```python
from build123d import *

# Parameters (mm, degrees)
SKETCH3_W           = 18.934254216
SKETCH3_H           = 5
BOSS_EXTRUDE1_DEPTH = 8
CUT_EXTRUDE1_REACH  = 24.954
SKETCH5_R           = 1.05
SKETCH4_W           = 5.27
SKETCH4_H           = 5
CUT_EXTRUDE2_DEPTH  = 2.9
SKETCH6_W           = 5.27
SKETCH6_H           = 5
CUT_EXTRUDE3_DEPTH  = 5.4
CUT_EXTRUDE5_REACH  = 15.365
CUT_EXTRUDE6_REACH  = 24.954
SKETCH10_R          = 1.7
CUT_EXTRUDE9_DEPTH  = 2
FILLET1_R           = 2.5
FILLET2_R           = 1.75
CUT_EXTRUDE7_REACH  = 15.365
SKETCH8_W           = 3.025341734
SKETCH8_H           = 1.75
CHAMFER1_SIZE       = 1


with BuildPart() as part:
    # Sketch3 → Boss-Extrude1 (new body)
    with BuildSketch(Plane.ZY):
        with Locations((0, 16.820132754)):
            Rectangle(SKETCH3_W, SKETCH3_H)
    extrude(amount=-BOSS_EXTRUDE1_DEPTH)

    # Sketch5 → Cut-Extrude1 (cut, up to next)
    with BuildSketch(Plane.ZY, mode=Mode.PRIVATE) as cut_extrude1_sk1:
        with Locations(Location((6.967127108, 16.820132754, 0), (0, 0, 270))):
            Circle(SKETCH5_R)
    cut_extrude1_tool1 = extrude(cut_extrude1_sk1.sketch, amount=-CUT_EXTRUDE1_REACH, mode=Mode.PRIVATE) & part.part
    # Sketch5 → Cut-Extrude1 (cut, up to next)
    with BuildSketch(Plane.ZY, mode=Mode.PRIVATE) as cut_extrude1_sk2:
        with Locations(Location((-6.967127108, 16.820132754, 0), (0, 0, 270))):
            Circle(SKETCH5_R)
    cut_extrude1_tool2 = extrude(cut_extrude1_sk2.sketch, amount=-CUT_EXTRUDE1_REACH, mode=Mode.PRIVATE) & part.part
    add(cut_extrude1_tool1.solids().sort_by_distance((0, 16.820133, 6.967127))[0], mode=Mode.SUBTRACT)
    add(cut_extrude1_tool2.solids().sort_by_distance((0, 16.820133, -6.967127))[0], mode=Mode.SUBTRACT)

    # Sketch4 → Cut-Extrude2 (cut)
    with BuildSketch(Plane.ZY):
        with Locations((6.832127108, 16.820132754)):
            Rectangle(SKETCH4_W, SKETCH4_H)
    extrude(amount=-CUT_EXTRUDE2_DEPTH, mode=Mode.SUBTRACT)

    # Sketch6 → Cut-Extrude3 (cut)
    with BuildSketch(Plane(origin=(8, 0, 0), x_dir=(0, 0, -1), z_dir=(1, 0, 0))):
        with Locations((6.832127108, 16.820132754)):
            Rectangle(SKETCH6_W, SKETCH6_H)
    extrude(amount=-CUT_EXTRUDE3_DEPTH, mode=Mode.SUBTRACT)

    # Sketch1 → Cut-Extrude5 (cut, up to next)
    with BuildSketch(Plane(origin=(0, 14.320132754, 0), x_dir=(-1, 0, 0), z_dir=(0, -1, 0)), mode=Mode.PRIVATE) as cut_extrude5_sk1:
        Polygon((3.959797975, 0), (0, -3.959797975), (-3.959797975, 0), (0, 3.959797975), align=None)
    cut_extrude5_tool1 = extrude(cut_extrude5_sk1.sketch, amount=-CUT_EXTRUDE5_REACH, mode=Mode.PRIVATE) & part.part
    add(cut_extrude5_tool1.solids().sort_by_distance((0, 14.320133, 0))[0], mode=Mode.SUBTRACT)

    # Sketch7 → Cut-Extrude6 (cut, up to next)
    with BuildSketch(Plane.ZY, mode=Mode.PRIVATE) as cut_extrude6_sk1:
        Polygon((-4.197127108, 17.820132754), (4.197127108, 17.820132754), (5.697127108, 19.320132754), (-5.697127108, 19.320132754), align=None)
    cut_extrude6_tool1 = extrude(cut_extrude6_sk1.sketch, amount=-CUT_EXTRUDE6_REACH, mode=Mode.PRIVATE) & part.part
    add(cut_extrude6_tool1.solids().sort_by_distance((0, 18.608034, 0))[0], mode=Mode.SUBTRACT)

    # Sketch10 → Cut-Extrude9 (cut)
    with BuildSketch(Plane(origin=(8, 0, 0), x_dir=(0, 0, -1), z_dir=(1, 0, 0))):
        with Locations(Location((-6.967127108, 16.820132754, 0), (0, 0, 90))):
            Circle(SKETCH10_R)
    extrude(amount=-CUT_EXTRUDE9_DEPTH, mode=Mode.SUBTRACT)

    # Mirror2: part across plane


with BuildPart() as part_1:
    add(part.part)
    add(part.part.mirror(Plane(origin=(0, 0, 0), x_dir=(0, 0, 1), z_dir=(1, 0, 0))))

    # Fillet1
    # the kernel refuses this fillet: 2.5 mm, written as the material it takes off along each edge
    with BuildSketch(Plane(origin=(3.35, 14.320132754, 9.467127108), x_dir=(0, 0, -1), z_dir=(-1, 0, 0)), Plane(origin=(-3.35, 19.320132754, 9.467127108), x_dir=(0, 0, -1), z_dir=(1, 0, 0))) as fillet1_piece_1:
        with BuildLine():
            CenterArc((FILLET1_R, -FILLET1_R), FILLET1_R, 90, 90)
            Line((0, -FILLET1_R), (0, 0))
            Line((0, 0), (FILLET1_R, 0))
        make_face()
    extrude(amount=17.6, mode=Mode.SUBTRACT)
    with BuildSketch(Plane(origin=(3.35, 19.320132754, 9.467127108), x_dir=(0, 0, -1), z_dir=(-1, 0, 0)), Plane(origin=(-3.35, 14.320132754, 9.467127108), x_dir=(0, 0, -1), z_dir=(1, 0, 0))) as fillet1_piece_2:
        with BuildLine():
            CenterArc((FILLET1_R, FILLET1_R), FILLET1_R, 180, 90)
            Line((0, FILLET1_R), (0, 0))
            Line((0, 0), (FILLET1_R, 0))
        make_face()
    extrude(amount=17.6, mode=Mode.SUBTRACT)
    with BuildSketch(Plane(origin=(-8.85, 14.320132754, -9.467127108), x_dir=(0, 0, 1), z_dir=(1, 0, 0))) as fillet1_piece_3:
        with BuildLine():
            CenterArc((FILLET1_R, -FILLET1_R), FILLET1_R, 90, 90)
            Line((0, -FILLET1_R), (0, 0))
            Line((0, 0), (FILLET1_R, 0))
        make_face()
    extrude(amount=17.7, mode=Mode.SUBTRACT)
    with BuildSketch(Plane(origin=(-8.85, 19.320132754, -9.467127108), x_dir=(0, 0, 1), z_dir=(1, 0, 0))) as fillet1_piece_4:
        with BuildLine():
            CenterArc((FILLET1_R, FILLET1_R), FILLET1_R, 180, 90)
            Line((0, FILLET1_R), (0, 0))
            Line((0, 0), (FILLET1_R, 0))
        make_face()
    extrude(amount=17.7, mode=Mode.SUBTRACT)

    # Fillet2
    # the kernel refuses this fillet: 1.75 mm, written as the material it takes off along each edge
    with BuildSketch(Plane(origin=(2.9, 14.320132754, 4.197127108), x_dir=(0, 0, -1), z_dir=(-1, 0, 0))) as fillet2_piece_1:
        with BuildLine():
            CenterArc((FILLET2_R, -FILLET2_R), FILLET2_R, 90, 90)
            Line((0, -FILLET2_R), (0, 0))
            Line((0, 0), (FILLET2_R, 0))
        make_face()
    extrude(amount=5.8, mode=Mode.SUBTRACT)
    with BuildSketch(Plane(origin=(2.9, 17.820132754, 4.197127108), x_dir=(0, 0, -1), z_dir=(-1, 0, 0))) as fillet2_piece_2:
        with BuildLine():
            CenterArc((FILLET2_R, FILLET2_R), FILLET2_R, 180, 90)
            Line((0, FILLET2_R), (0, 0))
            Line((0, 0), (FILLET2_R, 0))
        make_face()
    extrude(amount=5.8, mode=Mode.SUBTRACT)
    with BuildSketch(Plane(origin=(12.375, 14.320132754, -4.197127108), x_dir=(0, 0, 1), z_dir=(-1, 0, 0)), Plane(origin=(2.6, 17.820132754, -4.197127108), x_dir=(0, 0, 1), z_dir=(1, 0, 0))) as fillet2_piece_3:
        with BuildLine():
            CenterArc((FILLET2_R, FILLET2_R), FILLET2_R, 180, 90)
            Line((0, FILLET2_R), (0, 0))
            Line((0, 0), (FILLET2_R, 0))
        make_face()
    extrude(amount=9.775, mode=Mode.SUBTRACT)
    with BuildSketch(Plane(origin=(-12.375, 14.320132754, -4.197127108), x_dir=(0, 0, 1), z_dir=(1, 0, 0)), Plane(origin=(-2.6, 17.820132754, -4.197127108), x_dir=(0, 0, 1), z_dir=(-1, 0, 0))) as fillet2_piece_4:
        with BuildLine():
            CenterArc((FILLET2_R, -FILLET2_R), FILLET2_R, 90, 90)
            Line((0, -FILLET2_R), (0, 0))
            Line((0, 0), (FILLET2_R, 0))
        make_face()
    extrude(amount=9.775, mode=Mode.SUBTRACT)

    # Sketch8 → Cut-Extrude7 (cut, up to next)
    with BuildSketch(Plane(origin=(0, 14.320132754, 0), x_dir=(1, 0, 0), z_dir=(0, 1, 0)), mode=Mode.PRIVATE) as cut_extrude7_sk1:
        with Locations((0, -3.322127108)):
            Rectangle(SKETCH8_W, SKETCH8_H)
    cut_extrude7_tool1 = extrude(cut_extrude7_sk1.sketch, amount=CUT_EXTRUDE7_REACH, mode=Mode.PRIVATE) & part_1.part
    add(cut_extrude7_tool1.solids().sort_by_distance((0, 14.320133, 3.322127))[0], mode=Mode.SUBTRACT)

    # Chamfer1
    # the kernel refuses this chamfer: 1 mm, written as the material it takes off along each edge
    with BuildSketch(Plane(origin=(0.305783613, 14.320132754, 4.265581587), x_dir=(-0.7068394360706736, -0.027495876610585612, 0.7068394360706735), z_dir=(-0.7071067811865476, 0, -0.7071067811865476))) as chamfer1_piece_1:
        Polygon((CHAMFER1_SIZE * 0.999621916911, CHAMFER1_SIZE * 0.0274958766106), (-CHAMFER1_SIZE * 0.0274958766106, CHAMFER1_SIZE * 0.999621916911), (0, 0), align=None)
    extrude(amount=6.032443332, mode=Mode.SUBTRACT)
    with BuildSketch(Plane(origin=(-0.305783613, 14.320132754, 4.265581587), x_dir=(0.7068394360706735, -0.027495876610585612, 0.7068394360706735), z_dir=(0.7071067811865476, 0, -0.7071067811865476))) as chamfer1_piece_2:
        Polygon((CHAMFER1_SIZE * 0.999621916911, -CHAMFER1_SIZE * 0.0274958766106), (-CHAMFER1_SIZE * 0.0274958766106, -CHAMFER1_SIZE * 0.999621916911), (0, 0), align=None)
    extrude(amount=6.032443332, mode=Mode.SUBTRACT)
    with BuildSketch(Plane(origin=(3.959797975, 14.320132754, 0), x_dir=(0.7068394360706735, -0.027495876610590834, -0.7068394360706735), z_dir=(-0.7071067811865476, 0, -0.7071067811865476))) as chamfer1_piece_3:
        Polygon((CHAMFER1_SIZE * 0.999621916911, -CHAMFER1_SIZE * 0.0274958766106), (-CHAMFER1_SIZE * 0.0274958766106, -CHAMFER1_SIZE * 0.999621916911), (0, 0), align=None)
    extrude(amount=5.6, mode=Mode.SUBTRACT)
    with BuildSketch(Plane(origin=(-3.959797975, 14.320132754, 0), x_dir=(-0.7068394360706735, -0.027495876610590834, -0.7068394360706735), z_dir=(0.7071067811865476, 0, -0.7071067811865476))) as chamfer1_piece_4:
        Polygon((CHAMFER1_SIZE * 0.999621916911, CHAMFER1_SIZE * 0.0274958766106), (-CHAMFER1_SIZE * 0.0274958766106, CHAMFER1_SIZE * 0.999621916911), (0, 0), align=None)
    extrude(amount=5.6, mode=Mode.SUBTRACT)
    with BuildSketch(Plane(origin=(-5.778252454, 14.320132754, 1.81845448), x_dir=(-0.7068394360706735, -0.027495876610585616, -0.7068394360706735), z_dir=(0.7071067811865476, 0, -0.7071067811865476))) as chamfer1_piece_5a_section:
        Polygon((CHAMFER1_SIZE * 0.999621916911, CHAMFER1_SIZE * 0.0274958766106), (-CHAMFER1_SIZE * 0.0274958766106, CHAMFER1_SIZE * 0.999621916911), (0, 0), align=None)
    chamfer1_piece_5a = extrude(amount=8.171682988, mode=Mode.PRIVATE)
    chamfer1_piece_5a = split(chamfer1_piece_5a, bisect_by=Plane(origin=(-4.192997285, 14.649926381, -0.23319931), z_dir=(-0.7071067811865476, 0, 0.7071067811865476)), keep=Keep.TOP, mode=Mode.PRIVATE)
    with BuildSketch(Plane(origin=(0.305783613, 14.320132754, 4.265581587), x_dir=(-0.7068394360706736, -0.027495876610585612, 0.7068394360706735), z_dir=(-0.7071067811865476, 0, -0.7071067811865476))) as chamfer1_piece_5b_section:
        Polygon((CHAMFER1_SIZE * 0.999621916911, CHAMFER1_SIZE * 0.0274958766106), (-CHAMFER1_SIZE * 0.0274958766106, CHAMFER1_SIZE * 0.999621916911), (0, 0), align=None)
    chamfer1_piece_5b = extrude(amount=8.60412632, mode=Mode.PRIVATE)
    chamfer1_piece_5b = split(chamfer1_piece_5b, bisect_by=Plane(origin=(-4.192997285, 14.649926381, 0.23319931), z_dir=(-0.7071067811865476, 0, -0.7071067811865476)), keep=Keep.TOP, mode=Mode.PRIVATE)
    chamfer1_piece_5 = chamfer1_piece_5a & chamfer1_piece_5b
    add(chamfer1_piece_5, mode=Mode.SUBTRACT)
    with BuildSketch(Plane(origin=(-0.305783613, 14.320132754, 4.265581587), x_dir=(0.7068394360706735, -0.027495876610585612, 0.7068394360706735), z_dir=(0.7071067811865476, 0, -0.7071067811865476))) as chamfer1_piece_6a_section:
        Polygon((CHAMFER1_SIZE * 0.999621916911, -CHAMFER1_SIZE * 0.0274958766106), (-CHAMFER1_SIZE * 0.0274958766106, -CHAMFER1_SIZE * 0.999621916911), (0, 0), align=None)
    chamfer1_piece_6a = extrude(amount=8.60412632, mode=Mode.PRIVATE)
    chamfer1_piece_6a = split(chamfer1_piece_6a, bisect_by=Plane(origin=(4.192997285, 14.649926381, 0.23319931), z_dir=(0.7071067811865476, 0, -0.7071067811865476)), keep=Keep.TOP, mode=Mode.PRIVATE)
    with BuildSketch(Plane(origin=(5.778252454, 14.320132754, 1.81845448), x_dir=(0.7068394360706736, -0.027495876610585605, -0.7068394360706736), z_dir=(-0.7071067811865476, 0, -0.7071067811865476))) as chamfer1_piece_6b_section:
        Polygon((CHAMFER1_SIZE * 0.999621916911, -CHAMFER1_SIZE * 0.0274958766106), (-CHAMFER1_SIZE * 0.0274958766106, -CHAMFER1_SIZE * 0.999621916911), (0, 0), align=None)
    chamfer1_piece_6b = extrude(amount=8.171682988, mode=Mode.PRIVATE)
    chamfer1_piece_6b = split(chamfer1_piece_6b, bisect_by=Plane(origin=(4.192997285, 14.649926381, -0.23319931), z_dir=(0.7071067811865476, 0, 0.7071067811865476)), keep=Keep.TOP, mode=Mode.PRIVATE)
    chamfer1_piece_6 = chamfer1_piece_6a & chamfer1_piece_6b
    add(chamfer1_piece_6, mode=Mode.SUBTRACT)
    with BuildSketch(Plane(origin=(3.959797975, 14.320132754, 0), x_dir=(0.7068394360706735, -0.027495876610590834, -0.7068394360706735), z_dir=(-0.7071067811865476, 0, -0.7071067811865476))) as chamfer1_piece_7a_section:
        Polygon((CHAMFER1_SIZE * 0.999621916911, -CHAMFER1_SIZE * 0.0274958766106), (-CHAMFER1_SIZE * 0.0274958766106, -CHAMFER1_SIZE * 0.999621916911), (0, 0), align=None)
    chamfer1_piece_7a = extrude(amount=8.171682988, mode=Mode.PRIVATE)
    chamfer1_piece_7a = split(chamfer1_piece_7a, bisect_by=Plane(origin=(0.23319931, 14.649926381, -4.192997285), z_dir=(-0.7071067811865476, 0, -0.7071067811865476)), keep=Keep.TOP, mode=Mode.PRIVATE)
    with BuildSketch(Plane(origin=(-3.959797975, 14.320132754, 0), x_dir=(-0.7068394360706735, -0.027495876610590834, -0.7068394360706735), z_dir=(0.7071067811865476, 0, -0.7071067811865476))) as chamfer1_piece_7b_section:
        Polygon((CHAMFER1_SIZE * 0.999621916911, CHAMFER1_SIZE * 0.0274958766106), (-CHAMFER1_SIZE * 0.0274958766106, CHAMFER1_SIZE * 0.999621916911), (0, 0), align=None)
    chamfer1_piece_7b = extrude(amount=8.171682988, mode=Mode.PRIVATE)
    chamfer1_piece_7b = split(chamfer1_piece_7b, bisect_by=Plane(origin=(-0.23319931, 14.649926381, -4.192997285), z_dir=(0.7071067811865476, 0, -0.7071067811865476)), keep=Keep.TOP, mode=Mode.PRIVATE)
    chamfer1_piece_7 = chamfer1_piece_7a & chamfer1_piece_7b
    add(chamfer1_piece_7, mode=Mode.SUBTRACT)


solid = part_1.part
```
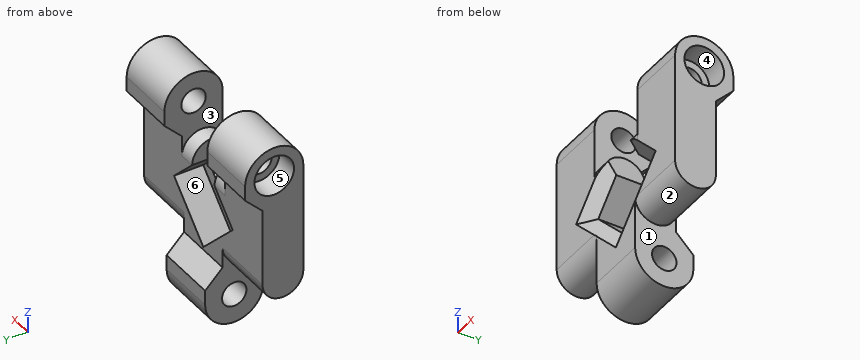
Geometry: final body of the model. Coordinates: model frame, mm. Face numbers are marked on the shaded views. A direction names the side the tool comes from. Give positions to 0.01 mm unless a question says otherwise; leave off trailing zeros. Write each loop counter-clockwise with the first axis right and the second up, starting at its lowest first coordinate (ties: lowest second). Pieces come first, ordered by that corner, then holes.
1. Section query A-A, the plane x = -2. Return loops of the section in (y, z).
2. Pin query (flat end, axial travel): P1, Ø2.5, axis at y = 16.82, z = 6.97, coming from the +X side; P2, Ø3, axis at x = -1.5, y = 16, coming from the +Z side; P3, Ø1.7, axis at y = 17, z = 7.5, coming from the -X side. Return the tip coordinate at first contact, or that it passes through.
3. Line query: probe 1 along X at (y, z) = (18.1, 7.5); probe 2 along Y at (x, z) = (-4.25, 7); probe 3 along Y at (x, z) = (-5, 2.5). Output: solid intervals per line, ascending.
4. Section query D-D, the plane z = -4.5. Return loops of the section in (x, y), then the cut area to 3 significant figures.
5. Draft query along X for the marked faces 1, 2 and 3. Return one class per face: released by +X, released by -X, zero draft, split by the parting line, or undercut.
6. Section query C-C, the plane y = 18.8. Return loops of the section in (x, z).
7. Reachability of the marked faces 4, 5 and 6 from +Z, -Z, +X, -X, +Y, -Y: full face, straight path, thin tool, end or side. Return the list, or none.
8. Section query B-B, the plane z = 0.25. Return loops of the section in (x, y).
Computed:
1. outline: (14.32, -6.97) arc R2.5 ccw to (19.32, -6.97) - (19.32, -5.7) - (17.82, -4.2) - (17.82, -1.96) - (15.32, -1.96) - (14.32, -3.37) - close; (14.47, 3.16) - (15.32, 1.96) - (17.82, 1.96) - (17.82, 2.45) arc R1.75 ccw to start; hole circle Ø2.1 at (16.82, -6.97)
2. P1: stops at x = 6
2. P2: stops at z = 9.45
2. P3: stops at x = -6
3. probe 1: x = -6 to -2.9, 2.9 to 6
3. probe 2: y = 14.32 to 15.77, 17.87 to 19.32
3. probe 3: y = 14.32 to 17.82
4. outline: (-2.6, 14.32) - (-0.87, 14.32) - (0, 14.94) - (0.87, 14.32) - (2.6, 14.32) - (2.6, 18.12) - (-2.6, 18.12) - close
4. area: 19.2 mm2
5. face 1: released by +X
5. face 2: zero draft
5. face 3: undercut
6. outline: (-8, 5.18) - (-2.9, 5.18) - (-2.9, 8.49) - (-8, 8.49) - close; (-2.6, -8.49) - (2.6, -8.49) - (2.6, -5.18) - (-2.6, -5.18) - close; (2.9, 5.18) - (8, 5.18) - (8, 8.49) - (2.9, 8.49) - close
7. face 4: +X
7. face 5: -X
7. face 6: +Y, -Y
8. outline: (-8, 14.32) - (-5.12, 14.32) - (-3.71, 15.32) - (-3.71, 17.82) - (-8, 17.82) - close; (3.71, 15.32) - (5.12, 14.32) - (8, 14.32) - (8, 17.82) - (3.71, 17.82) - close
